Check sheet for the modelled part. Datum: model origin and axes. Units: mm. A direction names the side the tool comes from. Give positions to 0.01 mm unless a question says otherwise; leave off trailing zeros. Order: outer loops, then holes, each group sorted by start corner. A loop starts at its lowest first (then second) coordinate and runs counter-clockwise, first axis right, second up.
```python
from build123d import *

# Parameters (mm, degrees)
SKETCH1_W           = 20
SKETCH1_H           = 30
SKETCH1_R           = 2.65
BOSS_EXTRUDE1_DEPTH = 3
SKETCH2_W           = 20
SKETCH2_H           = 10
BOSS_EXTRUDE2_DEPTH = 3
SKETCH3_W           = 1.8
SKETCH3_H           = 10
BOSS_EXTRUDE3_DEPTH = 10
FILLET1_R           = 5
CUT_EXTRUDE1_REACH  = 29.78
SKETCH4_R           = 1.5
CHAMFER1_SIZE       = 2
SKETCH5_W           = 20
SKETCH5_H           = 20
CUT_EXTRUDE2_DEPTH  = 10
SKETCH6_W           = 11
SKETCH6_H           = 10
BOSS_EXTRUDE4_DEPTH = 3.5
CUT_EXTRUDE3_DEPTH  = 3.5
SKETCH8_W           = 7.7
SKETCH8_H           = 31
SKETCH8_R           = 2.65
BOSS_EXTRUDE5_DEPTH = 14
SKETCH9_W           = 9
SKETCH9_H           = 21
CUT_EXTRUDE4_DEPTH  = 10


with BuildPart() as part:
    # Sketch1 → Boss-Extrude1 (new body)
    with BuildSketch(Plane.XY):
        Rectangle(SKETCH1_W, SKETCH1_H)
        with Locations((0, -10)):
            Circle(SKETCH1_R, mode=Mode.SUBTRACT)
        Circle(SKETCH1_R, mode=Mode.SUBTRACT)
    extrude(amount=BOSS_EXTRUDE1_DEPTH)

    # Sketch2 → Boss-Extrude2 (add)
    with BuildSketch(Plane.XY.offset(3)):
        with Locations((0, 10)):
            Rectangle(SKETCH2_W, SKETCH2_H)
    extrude(amount=BOSS_EXTRUDE2_DEPTH)

    # Sketch3 → Boss-Extrude3 (add)
    with BuildSketch(Plane.XY.offset(6)):
        with Locations((-6.15, 10)):
            Rectangle(SKETCH3_W, SKETCH3_H)
        with Locations((6.15, 10)):
            Rectangle(SKETCH3_W, SKETCH3_H)
    extrude(amount=BOSS_EXTRUDE3_DEPTH)

    # Fillet1
    fillet1_edges = [part.edges().sort_by_distance(p)[0] for p in [
        (6.15, 5, 16),
        (-6.15, 5, 16),
        (6.15, 15, 16),
        (-6.15, 15, 16),
    ]]
    fillet(fillet1_edges, radius=FILLET1_R - 0.0001)  # a hair under: the kernel refuses the full size

    # Cut-Extrude1: up to this face of the body (flat: up to its plane)
    cut_extrude1_end = Plane(part.part.faces().sort_by_distance((7.05, 10, 10.533268934))[0])
    # Sketch4 → Cut-Extrude1 (cut, up to the picked face)
    with BuildSketch(Plane.ZY.offset(7.05), mode=Mode.PRIVATE) as cut_extrude1_sk1:
        with Locations(Location((11, 10, 0), (0, 0, 270))):
            Circle(SKETCH4_R)
    cut_extrude1_tool1 = split(extrude(cut_extrude1_sk1.sketch, amount=-CUT_EXTRUDE1_REACH, mode=Mode.PRIVATE), bisect_by=cut_extrude1_end, keep=Keep.BOTH, mode=Mode.PRIVATE)
    add(cut_extrude1_tool1.solids().sort_by(Axis((-7.05, 10, 11), (1, 0, 0)))[0], mode=Mode.SUBTRACT)

    # Chamfer1
    chamfer1_edges = [part.edges().sort_by_distance(p)[0] for p in [
        (-7.05, 10, 6),
        (7.05, 10, 6),
    ]]
    chamfer(chamfer1_edges, length=CHAMFER1_SIZE)

    # Sketch5 → Cut-Extrude2 (cut)
    with BuildSketch(Plane.XY.offset(3)):
        with Locations((0, -5)):
            Rectangle(SKETCH5_W, SKETCH5_H)
    extrude(amount=-CUT_EXTRUDE2_DEPTH, mode=Mode.SUBTRACT)

    # Sketch6 → Boss-Extrude4 (add)
    with BuildSketch(Plane(origin=(10, 0, 0), x_dir=(0, 0, -1), z_dir=(1, 0, 0))):
        with Locations((-0.5, 10)):
            Rectangle(SKETCH6_W, SKETCH6_H)
    extrude(amount=BOSS_EXTRUDE4_DEPTH)

    # Sketch7 → Cut-Extrude3 (cut)
    with BuildSketch(Plane(origin=(13.5, 0, 0), x_dir=(0, 0, -1), z_dir=(1, 0, 0))):
        with BuildLine():
            Line((1.1, 8), (1.1, 12))
            ThreePointArc((1.1, 12), (2.5, 13.4), (3.9, 12))
            Line((3.9, 12), (3.9, 8))
            ThreePointArc((3.9, 8), (2.5, 6.6), (1.1, 8))
        make_face()
    extrude(amount=-CUT_EXTRUDE3_DEPTH, mode=Mode.SUBTRACT)

    # Sketch8 → Boss-Extrude5 (add)
    with BuildSketch(Plane.ZY.offset(10)):
        with Locations((3.85, -0.5)):
            Rectangle(SKETCH8_W, SKETCH8_H)
        with Locations((3.7, -11)):
            Circle(SKETCH8_R, mode=Mode.SUBTRACT)
    extrude(amount=BOSS_EXTRUDE5_DEPTH)

    # Sketch9 → Cut-Extrude4 (cut)
    with BuildSketch(Plane.XY.offset(7.7)):
        with Locations((-14.5, -5.5)):
            Rectangle(SKETCH9_W, SKETCH9_H)
    extrude(amount=-CUT_EXTRUDE4_DEPTH, mode=Mode.SUBTRACT)


solid = part.part
```
(1) Go/stop test with flat-tipped pins: P1, Ø5, axis at x = 6, y = 11.5, coming from the -Z side; P2, Ø8, axis at x = -6.5, z = 3, coming from the -Y side; P3, Ø4, axis at x = -19, y = -1, coming from the +Z side. Record where each tip stops, or that it passes through.
(2) Sectioned sample at D-D (z = 12). Enter the section's corners in (x, y).
(3) Tool access check on faces 1 (the face through (-3, 5, 3)), 2 (the face through (11.8, 13.4, -2.5)), 3 (the face through (5.25, 8.8, 9.8)). Record the directions out of +Z, -Z, +X, -X, +Y, -Y that give a thin tool (end or side, any length) a straight path to the whole face; none if there is none.
(4) Sectioned sample at B-B (y = -11). Enter the section's corners in (x, z).
(5) Sectioned sample at A-A (z = -2.5). Enter the section's corners in (x, y).
(6) Release check for a two-part mould opening along X. For faces 4 (the face through (-5, 15, 3)), 5 (the face through (-9.5, 10.1, 6)), 6 (the face through (10, 10.1, -0.8)) record: released by +X, released by -X, zero draft, split by the parting line, or undercut.
(7) Thickness scan on L1, parallel to Z at x = -20, y = -11; L2, parallel to Z at x = -6, y = 10; L3, parallel to Y at x = -7.5, z = 7. Record the ranges inside material, lowest first.
Values follow:
1. P1: stops at z = 0
1. P2: stops at y = 5
1. P3: stops at z = 7.7
2. outline: (-7.05, 5.1) - (-5.25, 5.1) - (-5.25, 8.88) - (-7.05, 8.88) - close; (-7.05, 11.12) - (-5.25, 11.12) - (-5.25, 14.9) - (-7.05, 14.9) - close; (5.25, 5.1) - (7.05, 5.1) - (7.05, 8.88) - (5.25, 8.88) - close; (5.25, 11.12) - (7.05, 11.12) - (7.05, 14.9) - (5.25, 14.9) - close
3. face 1: +Z, -Z, +X, -Y
3. face 2: +X, -X
3. face 3: +Z, +Y, -Y
4. outline: (-24, 0) - (-19, 0) - (-19, 1.05) - (-24, 1.05) - close; (-24, 6.35) - (-19, 6.35) - (-19, 7.7) - (-24, 7.7) - close
5. outline: (10, 5) - (13.5, 5) - (13.5, 6.6) - (10, 6.6) - close; (10, 13.4) - (13.5, 13.4) - (13.5, 15) - (10, 15) - close
6. face 4: zero draft
6. face 5: undercut
6. face 6: released by -X
7. L1: z = 0 to 1.05, 6.35 to 7.7
7. L2: z = 0 to 9.5, 12.5 to 16
7. L3: y = 5 to 15
